```python
from build123d import *

# Parameters (mm, degrees)
F0_R      = 94
F1_DEPTH  = 1.6
F2_R      = 0.6
F3_DEPTH  = 1.6
F5_DEPTH  = 1.6
F6_COUNT  = 8
F6_ANGLE  = 315
F8_DEPTH  = 1.6
F9_R      = 0.5
F9_R_2    = 5
F10_DEPTH = 1.6


with BuildPart() as f1:
    # F0 (on Top) → F1 (new body)
    with BuildSketch(Plane.XY):
        Circle(F0_R)
    extrude(amount=F1_DEPTH)

    # F2 (on Top) → F3 (cut, through all)
    with BuildSketch(Plane.XY):
        with Locations((0, 62.5)):
            Circle(F2_R)
        with Locations((-31.25, 54.1265877365)):
            Circle(F2_R)
        with Locations((-54.1265877365, 31.25)):
            Circle(F2_R)
        with Locations((-62.5, 0)):
            Circle(F2_R)
        with Locations((-54.1265877365, -31.25)):
            Circle(F2_R)
        with Locations((-31.25, -54.1265877365)):
            Circle(F2_R)
        with Locations((0, -62.5)):
            Circle(F2_R)
        with Locations((31.25, -54.1265877365)):
            Circle(F2_R)
        with Locations((54.1265877365, -31.25)):
            Circle(F2_R)
        with Locations((62.5, 0)):
            Circle(F2_R)
        with Locations((54.1265877365, 31.25)):
            Circle(F2_R)
        with Locations((31.25, 54.1265877365)):
            Circle(F2_R)
    extrude(amount=F3_DEPTH, mode=Mode.SUBTRACT)

    # F4 (on face) → F5 (cut, through all)
    with BuildSketch(Plane.XY.offset(1.6)):
        with BuildLine():
            Line((4.5, 79.5), (-4.5, 79.5))
            ThreePointArc((-4.5, 79.5), (-5.5606601718, 79.0606601718), (-6, 78))
            Line((-6, 78), (-6, 73))
            ThreePointArc((-6, 73), (-5.5606601718, 71.9393398282), (-4.5, 71.5))
            Line((-4.5, 71.5), (4.5, 71.5))
            ThreePointArc((4.5, 71.5), (5.5606601718, 71.9393398282), (6, 73))
            Line((6, 73), (6, 78))
            ThreePointArc((6, 78), (5.5606601718, 79.0606601718), (4.5, 79.5))
        make_face()
    f5 = extrude(amount=-F5_DEPTH, mode=Mode.SUBTRACT)

    # F6: F5 ×8 about axis
    f6_axis = Axis((0, 0, 1.6), (0, 0, 1))
    for i in range(1, F6_COUNT):
        add(f5.rotate(f6_axis, i * F6_ANGLE / (F6_COUNT - 1)), mode=Mode.SUBTRACT)

    # F7 (on face) → F8 (cut, through all)
    with BuildSketch(Plane(origin=(0, 0, 0), x_dir=(1, 0, 0), z_dir=(0, 0, -1))):
        with BuildLine():
            Line((-0.9, 43.4), (-19.9, 43.4))
            ThreePointArc((-19.9, 43.4), (-20.9606601718, 42.9606601718), (-21.4, 41.9))
            Line((-21.4, 41.9), (-21.4, 36.4))
            ThreePointArc((-21.4, 36.4), (-20.9606601718, 35.3393398282), (-19.9, 34.9))
            Line((-19.9, 34.9), (-0.9, 34.9))
            ThreePointArc((-0.9, 34.9), (0.1606601718, 35.3393398282), (0.6, 36.4))
            Line((0.6, 36.4), (0.6, 41.9))
            ThreePointArc((0.6, 41.9), (0.1606601718, 42.9606601718), (-0.9, 43.4))
        make_face()
    extrude(amount=-F8_DEPTH, mode=Mode.SUBTRACT)

    # F9 (on face) → F10 (cut, through all)
    with BuildSketch(Plane.XY.offset(1.6)):
        with Locations((-2, 20)):
            Circle(F9_R)
        with Locations((2, 20)):
            Circle(F9_R)
        Circle(F9_R_2)
    extrude(amount=-F10_DEPTH, mode=Mode.SUBTRACT)


solid = f1.part
```
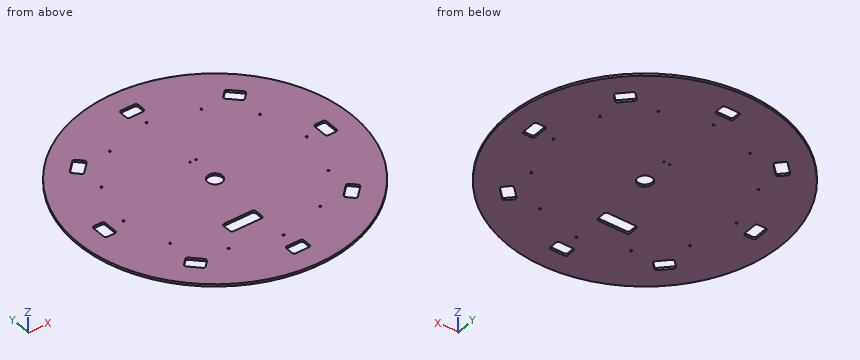
Model file for the job. Use its own axes, mm. Round coordinates to 2 decimals unless told otherwise and drop trailing zeros. Write each loop counter-clockwise with the first axis right and the second up, starting at its lowest first coordinate (ties: lowest second). Pieces come first, ordered by that corner, then holes. Notation, with made-up numbers: (33.5, -19) - (75.5, -19) arc R22 ccw to (75.5, 9) - close; hole circle Ø7 at (-8, -21.75). An arc over 180 degrees is marked (long way). One line per item, written item: value.
(1) Cut at A-A, the plane x = -17. Give the cut face in (y, z).
Values follow:
outline: (-92.45, 0) - (-43.4, 0) - (-43.4, 1.6) - (-92.45, 1.6) - close; (-34.9, 0) - (92.45, 0) - (92.45, 1.6) - (-34.9, 1.6) - close
(2) Wall check: probe 1 along Y at (x, z) = (56.5, 0.8); probe 2 along Y at (x, z) = (31.25, 0.3); probe 3 along Y at (x, z) = (-62.5, 0.85). Give the ranges that are in metal, low to high.
Values follow:
probe 1: y = -75.12 to -55.93, -48.01 to 48.01, 55.93 to 75.12
probe 2: y = -88.65 to -54.73, -53.53 to 53.53, 54.73 to 88.65
probe 3: y = -70.21 to -0.6, 0.6 to 70.21
(3) Cut at D-D, the plane y = 38.5. Give the cut face in (x, z).
Values follow:
outline: (-85.75, 0) - (85.75, 0) - (85.75, 1.6) - (-85.75, 1.6) - close
(4) Cut at C-C, the plane x = -36.5. Give the cut face in (y, z).
Values follow:
outline: (-86.62, 0) - (86.62, 0) - (86.62, 1.6) - (-86.62, 1.6) - close
(5) Drop flat-ended pins along their axis: P1, Ø0.8, axis at y = -76, z = 1, coming from the +X side; P2, Ø1, axis at x = 62.5, y = 0, coming from the +Z side; P3, Ø0.5, axis at x = 76, z = 1, coming from the +Y side; P4, Ø0.8, axis at x = 1.5, z = 0.5, coming from the -Y side. Give the stop position or say it passes through.
Values follow:
P1: stops at x = 55.86
P2: passes through
P3: stops at y = 55.66
P4: stops at y = -93.99
(6) Cut at B-B, the plane z = 1.35. Give the number of separate pieces and of enclosed holes in the cut face, plus the area to 3 significant figures.
Values follow:
separate pieces: 1
enclosed holes: 24
area: 26,700 mm²
